from build123d import *

# Parameters (mm, degrees)
F1_DEPTH = 39.878
F3_DEPTH = 58.42
F4_W     = 51.730605
F4_H     = 39.878
F5_DEPTH = 6.096
F6_R     = 4.89455
F7_DEPTH = 25.4


with BuildPart() as f1:
    # F0 (on Front) → F1 (new body)
    with BuildSketch(Plane.XZ):
        Polygon((37.552367, 65.042607), (-37.552367, 65.042607), (-75.104734, 0), (-37.552367, -65.042607), (37.552367, -65.042607), (75.104734, 0), align=None)
    extrude(amount=F1_DEPTH)

    # F2 (on face) → F3 (cut)
    with BuildSketch(Plane.XZ.offset(39.878)):
        Polygon((31.326826, 54.259654), (-31.326826, 54.259654), (-62.653652, 0), (-31.326826, -54.259654), (31.326826, -54.259654), (62.653652, 0), align=None)
    extrude(amount=-F3_DEPTH, mode=Mode.SUBTRACT)

    # F4 (on face) → F5 (join)
    with BuildSketch(Plane.XY.offset(65.042607)):
        with Locations((-0.68974, -19.939)):
            Rectangle(F4_W, F4_H)
    extrude(amount=F5_DEPTH)

    # F6 (on face) → F7 (cut)
    with BuildSketch(Plane.XY.offset(71.138607)):
        with Locations((0, -21.113751)):
            Circle(F6_R)
    extrude(amount=-F7_DEPTH, mode=Mode.SUBTRACT)


solid = f1.part
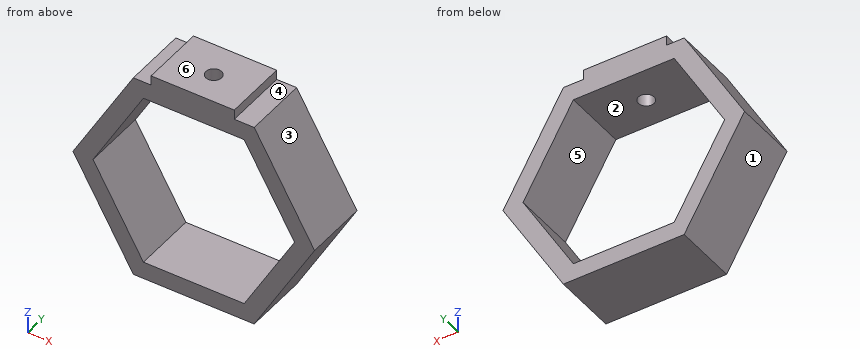
Input: part model. Units: mm. Frame: model coordinates. Face numbers are marked on the shaded views. A direction names the side the tool comes from. Round coordinates to 2 decimals unless told otherwise and drop trailing zeros. Write each loop counter-clockwise with the first axis right and the second up, starting at its lowest first coordinate (ties: lowest second). Pieces come first, ordered by that corner, then holes.
1) Cut plane D-D (y = -24). Return the cut outline in (x, z), then the cut area to 3 significant figures.
2) Ray query, L1, parallel to Z at x = -29, y = -29; L2, parallel to Y at x = 0, z = 59; L3, parallel to Z at x = 6, y = -34.5. Return the intervals inside material, ascending.
3) Reachability of the marked faces 4, 5 and 6 from +Z, -Z, +X, -X, +Y, -Y: full face, straight path, thin tool, end or side. Return the list, or none.
4) Cut plane B-B (y = -9). Return the cut outline in (x, z), then the cut area to 3 significant figures.
5) Cut plane A-A (x = 0). Return the cut outline in (y, z), then the cut area to 3 significant figures.
6) Draft query along Z for the marked faces 1, 2 and 3. Return one class per face: pulls with the +Z half, pulls with the -Z half, needs draft (parallel to the pull), parting line crosses it, or undercut.
7) Contact query for flat-ended pins moving along their axis: P1, Ø10, axis at x = 32, y = -15, coming from the +Z side; P2, Ø9, axis at x = 0, y = -21.11, coming from the +Z side; P3, Ø6, axis at y = -21.5, z = 39.5, coming from the -X side. Output: stop coordinate, or through.
8) Cut plane C-C (x = 61). Return the cut outline in (y, z).
Geometry says:
1. outline: (-75.1, 0) - (-37.55, -65.04) - (37.55, -65.04) - (75.1, 0) - (37.55, 65.04) - (25.18, 65.04) - (25.18, 71.14) - (3.95, 71.14) - (3.95, 54.26) - (31.33, 54.26) - (62.65, 0) - (31.33, -54.26) - (-31.33, -54.26) - (-62.65, 0) - (-31.33, 54.26) - (-3.95, 54.26) - (-3.95, 71.14) - (-26.56, 71.14) - (-26.56, 65.04) - (-37.55, 65.04) - close
1. area: 4,640 mm2
2. L1: z = -65.04 to -54.26, 54.26 to 65.04
2. L2: y = -39.88 to -26.01, -16.22 to 0
2. L3: z = -65.04 to -54.26, 54.26 to 71.14
3. face 4: +Z, +X, +Y, -Y
3. face 5: +Y, -Y
3. face 6: +Z, +X, -X, +Y, -Y
4. outline: (-75.1, 0) - (-37.55, -65.04) - (37.55, -65.04) - (75.1, 0) - (37.55, 65.04) - (25.18, 65.04) - (25.18, 71.14) - (-26.56, 71.14) - (-26.56, 65.04) - (-37.55, 65.04) - close; hole (-62.65, 0) - (-31.33, -54.26) - (31.33, -54.26) - (62.65, 0) - (31.33, 54.26) - (-31.33, 54.26) - close
4. area: 4,770 mm2
5. outline: (-39.88, -65.04) - (0, -65.04) - (0, -54.26) - (-39.88, -54.26) - close; (-39.88, 54.26) - (-26.01, 54.26) - (-26.01, 71.14) - (-39.88, 71.14) - close; (-16.22, 54.26) - (0, 54.26) - (0, 71.14) - (-16.22, 71.14) - close
5. area: 938 mm2
6. face 1: pulls with the -Z half
6. face 2: undercut
6. face 3: pulls with the +Z half
7. P1: stops at z = 65.04
7. P2: stops at z = -54.26
7. P3: stops at x = -54.03
8. outline: (-39.88, -24.43) - (0, -24.43) - (0, -2.86) - (-39.88, -2.86) - close; (-39.88, 2.86) - (0, 2.86) - (0, 24.43) - (-39.88, 24.43) - close
